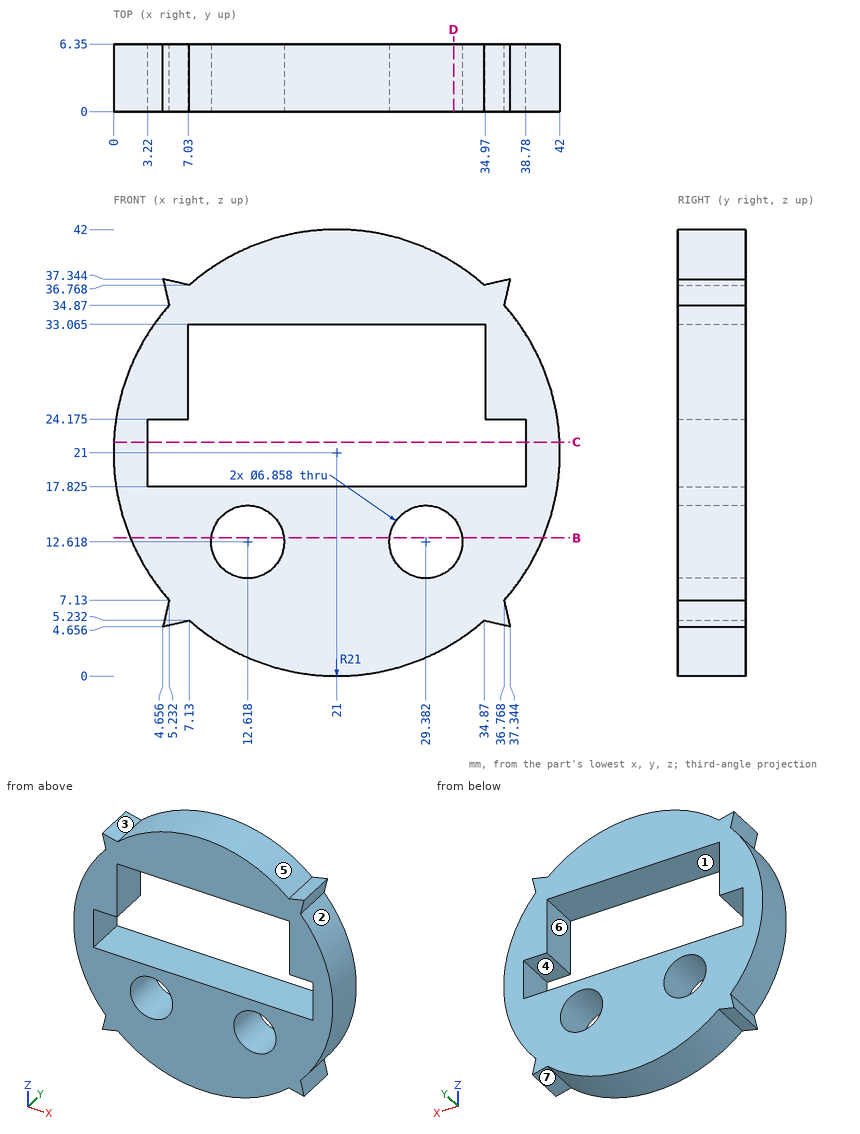
Study the drawing (mm; zero at the part's minimum x, y, z) and answer. A direction names the side the tool comes from. Give positions to 0.01 mm unless a question says otherwise; leave off trailing zeros. Write each loop counter-clockwise with the first axis right and the second up, starting at its lowest first coordinate (ties: lowest second). Pieces come first, ordered by that corner, then holes.
(1) The part is cut by section B-B on z = 13. Write down the section's boundary in (x, y).
Final values:
outline: (1.58, 0) - (9.21, 0) - (9.21, 6.35) - (1.58, 6.35) - close; (16.03, 0) - (25.97, 0) - (25.97, 6.35) - (16.03, 6.35) - close; (32.79, 0) - (40.42, 0) - (40.42, 6.35) - (32.79, 6.35) - close
(2) Which of the six approach directions +Z, -Z, +X, -X, +Y, -Y give full straight-line access (tool end or side, diameter ignored) to the marked faces 1, 2 and 3?
Final values:
face 1: +Y, -Y
face 2: +X, +Y, -Y
face 3: +Z, +Y, -Y
(3) Straight lines are drawn through the part: line 1 (X direction, y = 5.75, z = 13.5) (1 decimal); line 2 (Z direction, x = 21, y = 4.5) (1 decimal); line 3 (Z direction, x = 10, y = 5.5) (1 decimal). For each, find the intervals that lie inside material, in ascending order.
Final values:
line 1: x = 1.4 to 9.3, 15.9 to 26.1, 32.7 to 40.6
line 2: z = 0 to 17.8, 33.1 to 42
line 3: z = 3.1 to 10.4, 14.8 to 17.8, 33.1 to 38.9
(4) Flat-ended cylindrical pins translate along their axes: pin 1 Ø2 at (x, y) = (8.5, 3) entering from +Z; pin 2 Ø1.9 at (x, y) = (5.5, 2) entering from -Z; pin 3 Ø3 at (x, y) = (27.5, 3.5) entering from -Z. Find the tip coordinate at first contact, or state that the pin passes through.
Final values:
pin 1: stops at z = 38.57
pin 2: stops at z = 4.66
pin 3: stops at z = 0.6
(5) The mould has two halves that part along Z. Classify the marked faces 4, 5, 6 and 7: pulls with the +Z half, pulls with the -Z half, needs draft (parallel to the pull), parting line crosses it, or undercut.
Final values:
face 4: undercut
face 5: pulls with the +Z half
face 6: undercut
face 7: pulls with the -Z half
(6) The part is cut by section C-C on z = 22. Write down the section's boundary in (x, y), plus the area to 3 significant figures.
Final values:
outline: (0.02, 0) - (3.22, 0) - (3.22, 6.35) - (0.02, 6.35) - close; (38.78, 0) - (41.98, 0) - (41.98, 6.35) - (38.78, 6.35) - close
area: 40.6 mm2
(7) The part is cut by section D-D on x = 32. Count the separate pieces of the cut face and the enclosed holes in it, plus the area to 3 significant figures.
Final values:
separate pieces: 3
enclosed holes: 0
area: 102 mm2
